For this review, take the finished solid that the model builds, in its own axes (mm). Coordinates: 2 decimals unless noted, no trailing zeros. Write each loop counter-clockwise with the first axis right and the second up, starting at its lowest first coordinate (ties: lowest second). Pieces come first, ordered by that corner, then holes.
1) We need section A-A on x = 0. Write out the cut boundary in (y, z), then the cut area to 3 significant figures.
2) Mouldability with a two-part tool opening along X and no side actions: class faces 1 (the face through (-0.83, -0.99, 3.76)), 2 (the face through (4.91, 4.01, -1.55)), 3 (the face through (-0.1, 3, 3.4)), 4 (the face through (-3, -2, 2)) as pulls with the +X half, pulls with the -X half, needs draft (parallel to the pull), parting line crosses it, or undercut.
3) Insertion check: P1, Ø2, axis at x = -2, y = 1, coming from the -Z side; P2, Ø6, axis at x = 0, z = 0, coming from the -Y side; P3, Ø3, axis at x = 14, z = -8, coming from the -Y side. Each pin has a flat end and moves straight along its axis. Give the tip position at first contact, or say it passes through.
4) To check wall thickness, follow line 1 along Z through (x, y) = (0, 4.45); line 2 along Y through (x, z) = (-1, 15); line 3 along Z through (x, y) = (0, -1.35). State the ranges of each line that lie inside material, in increasing order.
5) We need section B-B on z = 0. Write out the cut boundary in (x, y), then the cut area to 3 significant figures.
6) We need section D-D on x = 14. Write out the cut boundary in (y, z).
7) We need section C-C on y = -0.5. Write out the cut boundary in (x, z), then the cut area to 3 significant figures.
Autodesk Inventor part; units mm, degrees
ref_plane "YZ Plane" through (0, 0, 0) normal (1, 0, 0) x (0, 1, 0)
ref_plane "XZ Plane" through (0, 0, 0) normal (0, 1, 0) x (-1, 0, 0)
ref_plane "XY Plane" through (0, 0, 0) normal (0, 0, 1) x (1, 0, 0)
sketch "Boceto1" plane through (0, 0, 0) normal (0, 1, 0) x (-1, 0, 0)
  circle A0 centre (0, 0) radius 21.5
  circle A1 centre (0, 0) radius 3.05
  dimension "d0" = 43
  dimension "d1" = 6.1
extrude "Extrusión1" add sketch "Boceto1" along normal blind 5
sketch "Boceto2" plane through (0, 5, 0) normal (0, 1, 0) x (1, 0, 0)
  circle A0 centre (0, 0) radius 5.15
  dimension "d4" = 10.3
extrude "Extrusión2" cut sketch "Boceto2" against normal blind 2
sketch "Boceto5" plane through (0, 0, 0) normal (0, -1, 0) x (1, 0, 0)
  circle A0 centre (0, 0) radius 3.85
  circle A1 centre (0, 0) radius 3.05
  dimension "d9" = 7.7
extrude "Extrusión3" add sketch "Boceto5" along normal blind 2
properties part number "Pulley Top"
Result:
1. outline: (-2, -3.85) - (0, -3.85) - (0, -21.5) - (5, -21.5) - (5, -5.15) - (3, -5.15) - (3, -3.05) - (-2, -3.05) - close; (-2, 3.05) - (3, 3.05) - (3, 5.15) - (5, 5.15) - (5, 21.5) - (0, 21.5) - (0, 3.85) - (-2, 3.85) - close
1. area: 179 mm2
2. face 1: parting line crosses it
2. face 2: undercut
2. face 3: undercut
2. face 4: needs draft
3. P1: stops at z = -21.48
3. P2: passes through
3. P3: stops at y = 0
4. line 1: z = -21.5 to -5.15, 5.15 to 21.5
4. line 2: y = 0 to 5
4. line 3: z = -3.85 to -3.05, 3.05 to 3.85
5. outline: (-21.5, 0) - (-3.85, 0) - (-3.85, -2) - (-3.05, -2) - (-3.05, 3) - (-5.15, 3) - (-5.15, 5) - (-21.5, 5) - close; (3.05, -2) - (3.85, -2) - (3.85, 0) - (21.5, 0) - (21.5, 5) - (5.15, 5) - (5.15, 3) - (3.05, 3) - close
5. area: 179 mm2
6. outline: (0, -16.32) - (5, -16.32) - (5, 16.32) - (0, 16.32) - close
7. outline: circle Ø7.7 at (0, 0); hole circle Ø6.1 at (0, 0)
7. area: 17.3 mm2
